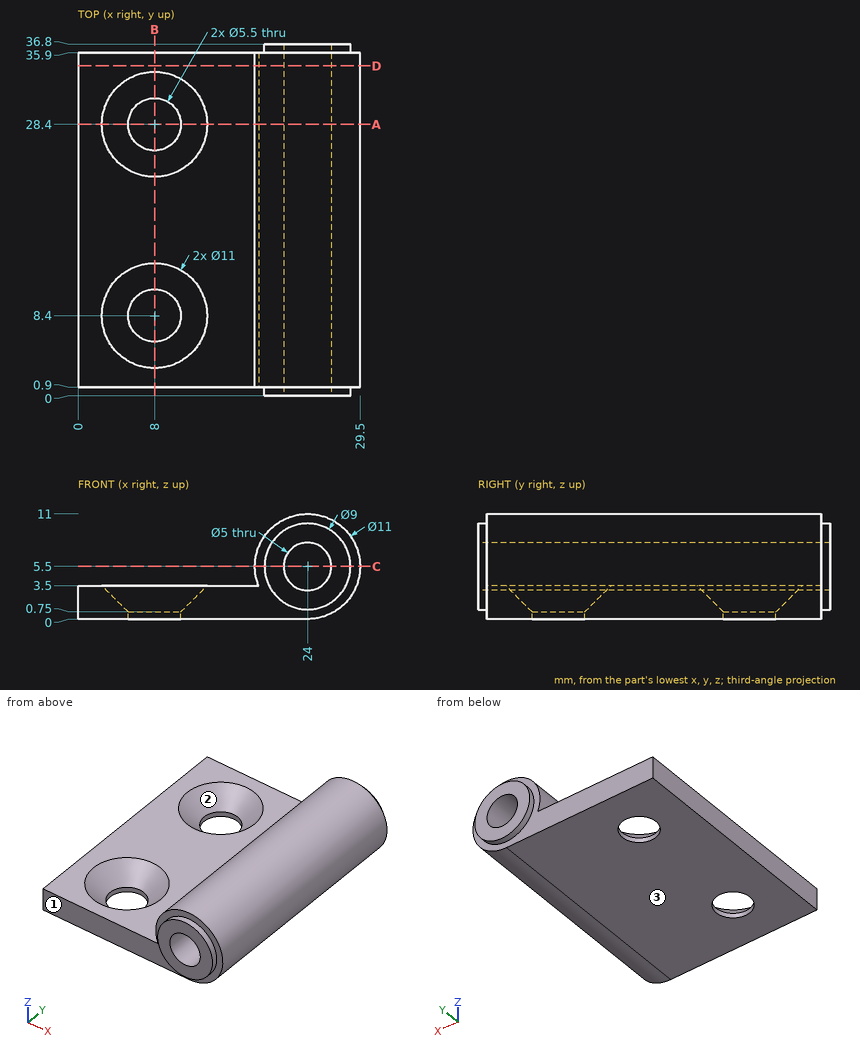
Study the drawing (mm; zero at the part's minimum x, y, z) and answer. Round coordinates to 2 decimals unless told otherwise and drop trailing zeros. Write each loop counter-clockwise with the first axis right and the second up, starting at its lowest first coordinate (ties: lowest second). Pieces come first, ordered by that corner, then holes.
1) A cutting plane is placed at B-B (x = 8). Give the vertices of the cut face in (y, z).
2) A cutting plane is placed at D-D (y = 34.5). Give the vertices of the cut face in (x, z).
3) Straight lines are drawn through the part: line 1 (Y direction, x = 8, z = 0.45); line 2 (Y direction, x = 11, z = 2.5); line 3 (Z direction, x = 24, y = 11.5). For each, find the intervals that lie inside material, in ascending order.
4) The mould has two halves that part along Y. Classify the marked faces 1, 2 and 3: pulls with the +Y half, pulls with the -Y half, needs draft (parallel to the pull), parting line crosses it, or undercut.
5) Given pin 1 Ø9.5 at (x, y) = (7.5, 12.5) entering from +Z; pin 2 Ø2 at (y, z) = (5, 3) entering from +X; pin 3 Ø6 at (y, z) = (26, 9.5) entering from -X, each flat-ended and moving along its own axis, determine where each tip first touches the part or whether it passes through.
6) A cutting plane is placed at C-C (z = 5.5). Give the vertices of the cut face in (x, y).
7) A cutting plane is placed at A-A (y = 28.4). Give the vertices of the cut face in (x, z), plus the area to 3 significant figures.
Completed:
1. outline: (0.9, 0) - (5.65, 0) - (5.65, 0.75) - (2.9, 3.5) - (0.9, 3.5) - close; (11.15, 0) - (25.65, 0) - (25.65, 0.75) - (22.9, 3.5) - (13.9, 3.5) - (11.15, 0.75) - close; (31.15, 0) - (35.9, 0) - (35.9, 3.5) - (33.9, 3.5) - (31.15, 0.75) - close
2. outline: (0, 0) - (24, 0) arc R5.5 ccw (long way) to (18.88, 3.5) - (0, 3.5) - close; hole circle Ø5 at (24, 5.5)
3. line 1: y = 0.9 to 5.65, 11.15 to 25.65, 31.15 to 35.9
3. line 2: y = 0.9 to 5.05, 11.75 to 25.05, 31.75 to 35.9
3. line 3: z = 0 to 3, 8 to 11
4. face 1: pulls with the -Y half
4. face 2: undercut
4. face 3: needs draft
5. pin 1: stops at z = 3.5
5. pin 2: stops at x = 29.29
5. pin 3: stops at x = 18.59
6. outline: (18.5, 0.9) - (19.5, 0.9) - (19.5, 0) - (21.5, 0) - (21.5, 36.8) - (19.5, 36.8) - (19.5, 35.9) - (18.5, 35.9) - close; (26.5, 0) - (28.5, 0) - (28.5, 0.9) - (29.5, 0.9) - (29.5, 35.9) - (28.5, 35.9) - (28.5, 36.8) - (26.5, 36.8) - close
7. outline: (0, 0) - (5.25, 0) - (5.25, 0.75) - (2.5, 3.5) - (0, 3.5) - close; (10.75, 0) - (24, 0) arc R5.5 ccw (long way) to (18.88, 3.5) - (13.5, 3.5) - (10.75, 0.75) - close; hole circle Ø5 at (24, 5.5)
7. area: 120 mm2
